from build123d import *

# Parameters (mm, degrees)
ESQUISSE1_R                  = 6
ESQUISSE1_R_2                = 4
BOSS_EXTRU_1_DEPTH           = 3
ENL_V_START                  = -3
ENL_V_MAT_EXTRU_1_DEPTH      = 3
R_P_TITION_CIRCULAIRE1_COUNT = 25


with BuildPart() as part:
    # Esquisse1 → Boss.-Extru.1 (new body)
    with BuildSketch(Plane.XY):
        Circle(ESQUISSE1_R)
        Circle(ESQUISSE1_R_2, mode=Mode.SUBTRACT)
    extrude(amount=BOSS_EXTRU_1_DEPTH)

    # Esquisse2 → Enlèv. mat.-Extru.1 (cut)
    with BuildSketch(Plane.XY.offset(3).offset(ENL_V_START)):
        with BuildLine():
            Line((-1.642379627, 5.770839554), (-1.642202224, 5.770714571))
            Line((-1.642202224, 5.770714571), (-0.793081387, 5.17249337))
            Line((-0.793081387, 5.17249337), (-0.160864862, 5.997843154))
            ThreePointArc((-0.160864862, 5.997843154), (-0.908738318, 5.930783647), (-1.642379627, 5.770839554))
        make_face()
    enl_v_mat_extru_1 = extrude(amount=ENL_V_MAT_EXTRU_1_DEPTH, mode=Mode.SUBTRACT)

    # Répétition circulaire1: Enlèv. mat.-Extru.1 ×25 about axis
    r_p_tition_circulaire1_axis = Axis((0, 0, 0), (0, 0, 1))
    for i in range(1, R_P_TITION_CIRCULAIRE1_COUNT):
        add(enl_v_mat_extru_1.rotate(r_p_tition_circulaire1_axis, i * 360 / R_P_TITION_CIRCULAIRE1_COUNT), mode=Mode.SUBTRACT)


solid = part.part
Build history of the part. All positions in model axes, mm. A direction names the side the tool comes from. Round coordinates to 2 decimals unless told otherwise and drop trailing zeros. Write each loop counter-clockwise with the first axis right and the second up, starting at its lowest first coordinate (ties: lowest second). Pieces come first, ordered by that corner, then holes. Notation, with made-up numbers: M 75,41 L 125,41 A30 cw 125,65 Z; hole C -39.75,73.5 d10. An arc over 180 degrees is marked long. Answer as a JSON object with one key per item and string values. Group by question number.
(1) Flat gauge pins, fed straight in: pin 1 (1 mm diameter, centred on x = 1, z = 0.5, fed in from -Y); pin 2 (1.5 mm diameter, centred on y = 2, z = 2.5, fed in from -X). Where does each tip first touch, or does it go through?
(2) Cut at A-A (y = 2.5). Give the cut face in (x, z).
(3) Which spindle directions (+Z, -Z, +X, -X, +Y, -Y) get a long thin tool onto all of the face, cutting with end or side? Do faces 1 (the flat face through (5.54, 0.83, 1.48)), 2 (the flat face through (-3.992, -3.927, 1.479)), 3 (the cylindrical face through (-0.867, -3.905, 1.479)), 4 (the flat face through (-1.854, 5.284, 1.479)), 5 (the flat face through (-5.46, 1.27, 1.48)). Say none if no direction does.
(4) Drill centre lines: L1, parallel to X at y = -0.25, z = 1.8; L2, parallel to Y at x = 0, z = 1.75; L3, parallel to X at y = -3.5, z = 1.65. Where is each one in solid material? Low to high.
(5) Cut at B-B (x = 0). Give the cut face in (y, z), and give its area (3 significant figures).
(6) Mould opens along X. For faces 6 (the flat face through (2.266, 5.121, 1.479)), 7 (the flat face through (-1.4, 4.1, 3)), 8 (the flat face through (5.253, -1.94, 1.479)), 9 (the flat face through (-4.969, 2.583, 1.479)) say: pulls with the +X half, pulls with the -X half, needs draft (parallel to the pull), parting line crosses it, or undercut.
Responses:
{
 "1": {"pin 1": "stops at y = -5.93", "pin 2": "stops at x = -5.75"},
 "2": {"outline": "M -4.94,0 L -3.12,0 L -3.12,3 L -4.94,3 Z; M 3.12,0 L 4.72,0 L 4.72,3 L 3.12,3 Z"},
 "3": {"face 1": "+Z, -Z, +X", "face 2": "+Z, -Z, -Y", "face 3": "+Z, -Z", "face 4": "+Z, -Z, +Y", "face 5": "+Z, -Z, -X"},
 "4": {"L1": "x = -5.46 to -3.99, 3.99 to 5.28", "L2": "y = -5.37 to -4, 4 to 5.82", "L3": "x = -4.44 to -1.94, 1.94 to 4.68"},
 "5": {"outline": "M -5.37,0 L -4,0 L -4,3 L -5.37,3 Z; M 4,0 L 5.82,0 L 5.82,3 L 4,3 Z", "area": "9.56 mm2"},
 "6": {"face 6": "undercut", "face 7": "needs draft", "face 8": "pulls with the +X half", "face 9": "pulls with the -X half"}
}
